For this review, take the finished solid that the model builds, in its own axes (mm). A direction names the side the tool comes from. Coordinates: 2 decimals unless noted, no trailing zeros. Order: outer loops, then holes, each group sorted by start corner. A loop starts at its lowest first (then second) coordinate and runs counter-clockwise, first axis right, second up. Notation, with made-up numbers: (12.5, -4.5) -> (31.5, -4.5) arc R11 cw to (31.5, 14.5) -> close; hole circle Ø5 at (29.5, 5). An arc over 180 degrees is marked (long way). Return JSON: item names as keys, results as strings. Group by question number.
Item 1: Take a section at D-D (x = 8). Write out the cut boundary in (y, z), then the cut area to 3 significant figures.
Item 2: For line 1 along Y through (x, z) = (63.5, 59.25) (3 decimals); line 2 along Z through (x, y) = (63, -40); line 3 along X through (y, z) = (-26, -11.5), list the stretches that pass through material, from the lowest coordinate up.
Item 3: Take a section at A-A (z = 48). Write out the cut boundary in (x, y), then the cut area to 3 significant figures.
Item 4: Draft analysis for pull direction X (two halves, no side actions). For faces 4 (the flat face through (127, 3, 17)), 5 (the cylindrical face through (69.36, -16.275, 26.833)), 6 (the flat face through (63, 0, -13)), state which applies: +X half, -X half, draft (parallel to the pull), parting line (faces both ways), or undercut.
Item 5: Insertion check: pin 1 (6.5 mm diameter, centred on x = 69, z = -13.5, fed in from +Y); pin 2 (4 mm diameter, centred on x = 59.5, y = 5, fed in from -Z); pin 3 (8 mm diameter, centred on y = -5.5, z = 29.5, fed in from -X). Each pin has a flat end and moves straight along its axis. Give the tip position at first contact, or say it passes through.
Item 6: Take a section at C-C (x = 79.5). Write out the cut boundary in (y, z), then the cut area to 3 significant figures.
Item 7: Take a section at B-B (y = -36.5). Write out the cut boundary in (x, z) (3 decimals), then the cut area to 3 significant figures.
Item 8: Machinability: for faces 1 (the flat face through (98.045, -21.914, 32.198)), 2 (the flat face through (50.8, -22, -4)), 3 (the flat face through (76.2, -22, -5)), which of the approach directions +Z, -Z, +X, -X, +Y, -Y give a long, thin tool a straight path to every point of the face, cutting with its end or side? Answer none if there is none.
```python
from build123d import *

# Parameters (mm, degrees)
F0_R     = 12.7
F1_DEPTH = 44.45
F2_W     = 127
F2_H     = 63.5
F3_DEPTH = 12.7
F4_R     = 12.7
F5_DEPTH = 12.701
F7_DEPTH = 25.4


with BuildPart() as f1:
    # F0 (on Front) → F1 (new body)
    with BuildSketch(Plane.XZ):
        with BuildLine():
            Line((0, 12.7), (0, 0))
            Line((0, 0), (50.8, 0))
            Line((50.8, 0), (50.8, -8.89))
            Line((50.8, -8.89), (31.75, -8.89))
            Line((31.75, -8.89), (31.75, -21.59))
            Line((31.75, -21.59), (95.25, -21.59))
            Line((95.25, -21.59), (95.25, -8.89))
            Line((95.25, -8.89), (76.2, -8.89))
            Line((76.2, -8.89), (76.2, 0))
            Line((76.2, 0), (127, 0))
            Line((127, 0), (127, 12.7))
            Line((127, 12.7), (111.125, 12.7))
            Line((111.125, 12.7), (84.593426, 52.250173))
            ThreePointArc((84.593426, 52.250173), (63.5, 63.5), (42.406574, 52.250173))
            Line((42.406574, 52.250173), (15.875, 12.7))
            Line((15.875, 12.7), (0, 12.7))
        make_face()
        with Locations((63.5, 38.1)):
            Circle(F0_R, mode=Mode.SUBTRACT)
    extrude(amount=F1_DEPTH)

    # F2 (on face) → F3 (join)
    with BuildSketch(Plane(origin=(0, 0, 0), x_dir=(-1, 0, 0), z_dir=(0, 1, 0))):
        with Locations((-63.5, 31.75)):
            Rectangle(F2_W, F2_H)
    extrude(amount=F3_DEPTH)

    # F4 (on face) → F5 (cut, through all)
    with BuildSketch(Plane.XZ):
        with Locations((63.5, 38.1)):
            Circle(F4_R)
    extrude(amount=-F5_DEPTH, mode=Mode.SUBTRACT)

    # F6 (on face) → F7 (cut)
    with BuildSketch(Plane.XY.offset(63.5)):
        with BuildLine():
            Line((63.5, -22.225), (68.58, -22.225))
            ThreePointArc((68.58, -22.225), (63.5, -17.145), (58.42, -22.225))
            Line((58.42, -22.225), (63.5, -22.225))
        make_face()
        with BuildLine():
            ThreePointArc((58.42, -22.225), (63.5, -27.305), (68.58, -22.225))
            Line((68.58, -22.225), (63.5, -22.225))
            Line((63.5, -22.225), (58.42, -22.225))
        make_face()
    extrude(amount=-F7_DEPTH, mode=Mode.SUBTRACT)


solid = f1.part
```
Findings below:
{
 "1": {"outline": "(-44.45, 0) -> (12.7, 0) -> (12.7, 63.5) -> (0, 63.5) -> (0, 12.7) -> (-44.45, 12.7) -> close", "area": "1,370 mm2"},
 "2": {"line 1": "y = -44.45 to -27.305, -17.145 to 12.7", "line 2": "z = -21.59 to 25.41, 50.79 to 63.5", "line 3": "x = 31.75 to 95.25"},
 "3": {"outline": "(0, 0) -> (39.56, 0) -> (39.56, -44.45) -> (55.55, -44.45) -> (55.55, 12.7) -> (0, 12.7) -> close; (71.45, -44.45) -> (87.44, -44.45) -> (87.44, 0) -> (127, 0) -> (127, 12.7) -> (71.45, 12.7) -> close", "area": "2,830 mm2"},
 "4": {"face 4": "+X half", "face 5": "undercut", "face 6": "draft"},
 "5": {"pin 1": "stops at y = 0", "pin 2": "stops at z = 0", "pin 3": "stops at x = 24.46"},
 "6": {"outline": "(-44.45, -21.59) -> (0, -21.59) -> (0, -8.89) -> (-44.45, -8.89) -> close; (-44.45, 0) -> (12.7, 0) -> (12.7, 63.5) -> (0, 63.5) -> (0, 57.83) -> (-44.45, 57.83) -> close", "area": "3,940 mm2"},
 "7": {"outline": "(0, 0) -> (50.8, 0) -> (50.8, -8.89) -> (31.75, -8.89) -> (31.75, -21.59) -> (95.25, -21.59) -> (95.25, -8.89) -> (76.2, -8.89) -> (76.2, 0) -> (127, 0) -> (127, 12.7) -> (111.125, 12.7) -> (84.593, 52.25) arc R25.4 ccw to (42.407, 52.25) -> (15.875, 12.7) -> (0, 12.7) -> close; hole circle Ø25.4 at (63.5, 38.1)", "area": "5,190 mm2"},
 "8": {"face 1": "+Z, +X, -Y", "face 2": "-X, +Y, -Y", "face 3": "+X, +Y, -Y"}
}
